Read the model definition and answer for the solid it produces. Units are mm, in the model's axes. A direction names the side the tool comes from. Coordinates: 2 decimals unless noted, no trailing zeros. Order: outer loops, then holes, each group sorted by start corner. A loop starts at its lowest first (then second) coordinate and runs counter-clockwise, first axis right, second up. Notation, with made-up numbers: (32, 16) -> (47, 16) arc R30 ccw to (47, 41) -> close; hole circle Ø4 at (8.5, 81). An arc over 180 degrees is marked (long way). Use CSV: the item, a comma, the result in double quotes.
```python
from build123d import *

# Parameters (mm, degrees)
SKETCH1_R           = 3.5
BOSS_EXTRUDE1_DEPTH = 30
BOSS_EXTRUDE2_DEPTH = 50.8
SKETCH3_R           = 4
BOSS_EXTRUDE3_DEPTH = 10
CHAMFER1_SIZE       = 1
SKETCH4_W           = 30
SKETCH4_H           = 11
CUT_EXTRUDE1_DEPTH  = 95.850619397


with BuildPart() as part:
    # Sketch1 → Boss-Extrude1 (new body)
    with BuildSketch(Plane(origin=(0, 0, 0), x_dir=(1, 0, 0), z_dir=(0, 1, 0))):
        with BuildLine():
            Line((-10, 10), (10, 10))
            ThreePointArc((10, 10), (20, 0), (10, -10))
            Line((10, -10), (-10, -10))
            ThreePointArc((-10, -10), (-20, 0), (-10, 10))
        make_face()
        with Locations(Location((-10, 0, 0), (0, 0, 270))):
            Circle(SKETCH1_R, mode=Mode.SUBTRACT)
        with Locations(Location((10, 0, 0), (0, 0, 270))):
            Circle(SKETCH1_R, mode=Mode.SUBTRACT)
    extrude(amount=BOSS_EXTRUDE1_DEPTH)

    # Sketch2 → Boss-Extrude2 (add)
    with BuildSketch(Plane.XZ):
        with BuildLine():
            Line((-10, -5), (-65, -5))
            ThreePointArc((-65, -5), (-70, 0), (-65, 5))
            Line((-65, 5), (-10, 5))
            ThreePointArc((-10, 5), (-5, 0), (-10, -5))
        make_face()
    extrude(amount=BOSS_EXTRUDE2_DEPTH)

    # Sketch3 → Boss-Extrude3 (add)
    with BuildSketch(Plane.XZ.offset(50.8)):
        with Locations(Location((-10, 0, 0), (0, 0, 270))):
            Circle(SKETCH3_R)
    extrude(amount=BOSS_EXTRUDE3_DEPTH)

    # Chamfer1
    chamfer1_edges = [part.edges().sort_by_distance(p)[0] for p in [
        (-10, -60.8, 4),
    ]]
    chamfer(chamfer1_edges, length=CHAMFER1_SIZE)

    # Sketch4 → Cut-Extrude1 (cut, through all)
    with BuildSketch(Plane(origin=(0, 0, -10), x_dir=(-1, 0, 0), z_dir=(0, 0, -1))):
        with Locations((-15, 15.456720209)):
            Rectangle(SKETCH4_W, SKETCH4_H)
    extrude(amount=-CUT_EXTRUDE1_DEPTH, mode=Mode.SUBTRACT)


solid = part.part
```
Item 1: The mould has two halves that part along X. Classify faces 1 (the cylindrical face through (6.583, 4.909, -0.759)), 2 (the cylindrical face through (20, 25, 0)), 3 (the cylindrical face through (-13.905, -55.237, 0.867)): +X half, -X half, draft (parallel to the pull), parting line (faces both ways), or undercut.
Return value:
face 1,"undercut"
face 2,"+X half"
face 3,"parting line"
Item 2: Find section A-A, the plane z = 0. Give the number of separate pieces and of enclosed holes in the cut face, then the cut area to 3 significant figures.
Return value:
separate pieces,"3"
enclosed holes,"0"
area,"4,020 mm^2"
Item 3: Each of these flat-tipped pins is pushed along its axis until it touches: P1, Ø2, axis at y = -27.5, z = -2.5, coming from the -X side; P2, Ø2, axis at x = -36.5, z = 3.5, coming from the +Y side; P3, Ø8, axis at x = -51, y = -49, coming from the -Z side. Where does it stop, or does it pass through?
Return value:
P1,"stops at x = -69.77"
P2,"stops at y = 0"
P3,"stops at z = -5"
Item 4: Find section C-C, the plane z = 6.25. Give the vertices of the cut face in (x, y).
Return value:
outline,"(-17.81, 0) -> (17.81, 0) -> (17.81, 9.96) -> (0, 9.96) -> (0, 20.96) -> (17.81, 20.96) -> (17.81, 30) -> (-17.81, 30) -> close"
Item 5: A tool of negligible diameter and unlimited length cuts with its end or side. For faces 4 (the flat face through (6, 9.957, 0)), 5 (the cylindrical face through (-5, -25, 0)), 6 (the cylindrical face through (-20, 15, 0)), 7 (the flat face through (-10, 0, 0)), from which of +Z, -Z, +X, -X, +Y, -Y can it reach the whole face along a straight path? Write none if from no direction.
Return value:
face 4,"+Z, -Z, +X"
face 5,"+X, -Y"
face 6,"-X, +Y"
face 7,"+Y"
Item 6: Find section B-B, the plane x = -2. Give the vertices of the cut face in (y, z), then the cut area to 3 significant figures.
Return value:
outline,"(0, -10) -> (30, -10) -> (30, 10) -> (0, 10) -> close"
area,"600 mm^2"
Item 7: Straight lines are drawn through the part: line 1 along X through (y, z) = (26, 0); line 2 along Z through (x, y) = (10, 23.5); line 3 along Y through (x, z) = (5, 9.25). For each, find the intervals that lie inside material, in ascending order.
Return value:
line 1,"x = -20 to -13.5, -6.5 to 6.5, 13.5 to 20"
line 2,"z = -10 to -3.5, 3.5 to 10"
line 3,"y = 0 to 9.96, 20.96 to 30"
Item 8: Find section D-D, the plane y = -17.5. Give the vertices of the cut face in (x, z), then the cut area to 3 significant figures.
Return value:
outline,"(-65, -5) -> (-10, -5) arc R5 ccw to (-10, 5) -> (-65, 5) arc R5 ccw to start"
area,"629 mm^2"
